Work out the finished part from the listing and answer in its coordinate system (mm). A direction names the side the tool comes from. Round coordinates to 2 decimals unless told otherwise and drop trailing zeros. Loops run counter-clockwise (first coordinate to the right, second up) from the corner with the lowest first, then second, coordinate; pieces in that order, holes last. Notation, with made-up numbers: M 35.25,58.25 L 66.25,58.25 A18 cw 66.25,85.25 Z; hole C 28,-26 d7. An arc over 180 degrees is marked long. One line per item, written item: value.
```python
from build123d import *

# Parameters (mm, degrees)
SKETCH1_R           = 13.0175
SKETCH1_R_2         = 2.38125
BOSS_EXTRUDE1_DEPTH = 7.9375
SKETCH2_R           = 11.1125
SKETCH2_R_2         = 4.7625
CUT_EXTRUDE1_DEPTH  = 0.8128
SKETCH3_R           = 11.1125
SKETCH3_R_2         = 4.7625
CUT_EXTRUDE2_DEPTH  = 0.8128
SKETCH4_R           = 1.28905
CUT_EXTRUDE3_DEPTH  = 14.0175


with BuildPart() as part:
    # Sketch1 → Boss-Extrude1 (new body)
    with BuildSketch(Plane(origin=(0, 0, 0), x_dir=(1, 0, 0), z_dir=(0, 1, 0))):
        Circle(SKETCH1_R)
        Circle(SKETCH1_R_2, mode=Mode.SUBTRACT)
    extrude(amount=BOSS_EXTRUDE1_DEPTH)

    # Sketch2 → Cut-Extrude1 (cut)
    with BuildSketch(Plane(origin=(0, 7.9375, 0), x_dir=(1, 0, 0), z_dir=(0, 1, 0))):
        Circle(SKETCH2_R)
        Circle(SKETCH2_R_2, mode=Mode.SUBTRACT)
    extrude(amount=-CUT_EXTRUDE1_DEPTH, mode=Mode.SUBTRACT)

    # Sketch3 → Cut-Extrude2 (cut)
    with BuildSketch(Plane.XZ):
        Circle(SKETCH3_R)
        Circle(SKETCH3_R_2, mode=Mode.SUBTRACT)
    extrude(amount=-CUT_EXTRUDE2_DEPTH, mode=Mode.SUBTRACT)

    # Sketch4 → Cut-Extrude3 (cut, through all)
    with BuildSketch(Plane.XY):
        with Locations((0, 3.9624)):
            Circle(SKETCH4_R)
    extrude(amount=-CUT_EXTRUDE3_DEPTH, mode=Mode.SUBTRACT)


solid = part.part
```
1) The mould has two halves that part along Z. Classify faces 6 (the face through (-1.695, 3.913, -12.907)), 7 (the face through (10, 0, -6)), 8 (the face through (-3.78, 7.54, 2.9)): +Z half, -Z half, draft (parallel to the pull), parting line (faces both ways), or undercut.
Check values:
face 6: parting line
face 7: draft
face 8: undercut
2) Find section D-D (x = 10). Give the vertices of the cut face in (y, z).
Check values:
outline: M 0,-8.33 L 7.94,-8.33 L 7.94,-4.85 L 7.12,-4.85 L 7.12,4.85 L 7.94,4.85 L 7.94,8.33 L 0,8.33 L 0,4.85 L 0.81,4.85 L 0.81,-4.85 L 0,-4.85 Z
3) Find section B-B (z = 0). Give the vertices of the cut face in (x, y), then the cut area to 3 significant figures.
Check values:
outline: M -13.02,0 L -11.11,0 L -11.11,0.81 L -4.76,0.81 L -4.76,0 L -2.38,0 L -2.38,7.94 L -4.76,7.94 L -4.76,7.12 L -11.11,7.12 L -11.11,7.94 L -13.02,7.94 Z; M 2.38,0 L 4.76,0 L 4.76,0.81 L 11.11,0.81 L 11.11,0 L 13.02,0 L 13.02,7.94 L 11.11,7.94 L 11.11,7.12 L 4.76,7.12 L 4.76,7.94 L 2.38,7.94 Z
area: 148 mm2
4) For faces 1 (the face through (10, 7.938, -6)), 2 (the face through (-3.78, 0.4, -2.9)), 3 (the face through (2, 0, 2)), 4 (the face through (0, 7.125, 5)), 5 (the face through (-0.279, 2.704, -7.434)), determine the directions among +Z, -Z, +X, -X, +Y, -Y from which every point of the face is accessible in a straight line to the end or side of a thin tool.
Check values:
face 1: +Z, -Z, +X, -X, +Y
face 2: -Y
face 3: +Z, -Z, +X, -X, -Y
face 4: +Y
face 5: -Z
5) Find the intervals of material crossed by probe 1 along X at (y, z) = (7.45, 0); probe 2 along Z at (x, y) = (0, 6), in increasing order. Write a range as from..to.
Check values:
probe 1: -13.02..-11.11, -4.76..-2.38, 2.38..4.76, 11.11..13.02
probe 2: -13.02..-2.38, 2.38..13.02
6) Find section A-A (x = 0). Give the vertices of the cut face in (y, z).
Check values:
outline: M 0,-13.02 L 2.67,-13.02 L 2.67,-2.38 L 0,-2.38 L 0,-4.76 L 0.81,-4.76 L 0.81,-11.11 L 0,-11.11 Z; M 0,2.38 L 7.94,2.38 L 7.94,4.76 L 7.12,4.76 L 7.12,11.11 L 7.94,11.11 L 7.94,13.02 L 0,13.02 L 0,11.11 L 0.81,11.11 L 0.81,4.76 L 0,4.76 Z; M 5.25,-13.02 L 7.94,-13.02 L 7.94,-11.11 L 7.12,-11.11 L 7.12,-4.76 L 7.94,-4.76 L 7.94,-2.38 L 5.25,-2.38 Z
7) Find section C-C (y = 0.5). Give the vertices of the cut face in (x, z) (1 decimal), then the cut area to 3 significant figures.
Check values:
outline: C 0,0 d26; C 0,0 d9.5; hole C 0,0 d22.2; hole C 0,0 d4.8
area: 198 mm2
8) Each of these flat-tipped pins is pushed along its axis until it touches: pin 1 (1.5 mm diameter, centred on y = 2.5, z = -2.5, fed in from +X); pin 2 (2 mm diameter, centred on x = -2, y = 4.5, fed in from +Z); pin 3 (2.5 mm diameter, centred on x = 0, y = 3.96, fed in from -Z); pin 4 (4 mm diameter, centred on x = 0, z = 0, fed in from -Y). Where does it stop, or does it pass through?
Check values:
pin 1: x = 12.9
pin 2: z = 12.98
pin 3: z = 2.03
pin 4: through
